```python
from build123d import *

# Parameters (mm, degrees)
F0_W     = 76.2
F0_H     = 76.2
F1_DEPTH = 584.2
F3_DEPTH = 38.1
F4_W     = 38.1
F4_H     = 38.1
F5_DEPTH = 38.1
F6_W     = 25.4
F6_H     = 114.3
F7_DEPTH = 76.201


with BuildPart() as f1:
    # F0 (on Top) → F1 (new body)
    with BuildSketch(Plane.XY):
        Rectangle(F0_W, F0_H)
    extrude(amount=F1_DEPTH)

    # F2 (on face) → F3 (join)
    with BuildSketch(Plane.XY.offset(584.2)):
        Polygon((-19.05, -19.05), (19.05, -19.05), (-19.05, 19.05), align=None)
        Polygon((-19.05, 19.05), (19.05, -19.05), (19.05, 19.05), align=None)
    extrude(amount=F3_DEPTH)

    # F4 (on face) → F5 (join)
    with BuildSketch(Plane(origin=(0, 0, 0), x_dir=(1, 0, 0), z_dir=(0, 0, -1))):
        Rectangle(F4_W, F4_H)
    extrude(amount=F5_DEPTH)

    # F6 (on face) → F7 (cut, through all)
    with BuildSketch(Plane(origin=(0, 38.1, 0), x_dir=(-1, 0, 0), z_dir=(0, 1, 0))):
        with Locations((0, 292.1)):
            Rectangle(F6_W, F6_H)
    extrude(amount=-F7_DEPTH, mode=Mode.SUBTRACT)


solid = f1.part
```
For this review, take the finished solid that the model builds, in its own axes (mm). A direction names the side the tool comes from. Round coordinates to 2 decimals unless told otherwise and drop trailing zeros. Order: outer loops, then holes, each group sorted by start corner. A loop starts at its lowest first (then second) coordinate and runs counter-clockwise, first axis right, second up.
Q1. We need section D-D, the plane x = -29. Give the boundary of the cut face in (y, z), plus the area to 3 significant figures.
Findings below:
outline: (-38.1, 0) - (38.1, 0) - (38.1, 584.2) - (-38.1, 584.2) - close
area: 44,500 mm2
Q2. Mouldability with a two-part tool opening along Z and no side actions: class faces 4 (the flat face through (0, 0, 622.3)), 5 (the flat face through (19.05, 0, -19)), 6 (the flat face through (-12.7, 1, 291)), 7 (the flat face through (0, 0, -38.1)) as pulls with the +Z half, pulls with the -Z half, needs draft (parallel to the pull), parting line crosses it, or undercut.
Findings below:
face 4: pulls with the +Z half
face 5: needs draft
face 6: undercut
face 7: pulls with the -Z half
Q3. Insertion check: P1, Ø11.5, axis at y = 4.5, z = -17, coming from the +X side; P2, Ø1, axis at x = -22.5, y = 6.5, coming from the -Z side; P3, Ø19, axis at y = -4.5, z = -12.5, coming from the -X side. Each pin has a flat end and moves straight along its axis. Give the tip position at first contact, or say it passes through.
Findings below:
P1: stops at x = 19.05
P2: stops at z = 0
P3: stops at x = -19.05
Q4. We need section C-C, the plane y = 5.5. Give the boundary of the cut face in (x, z).
Findings below:
outline: (-38.1, 0) - (-19.05, 0) - (-19.05, -38.1) - (19.05, -38.1) - (19.05, 0) - (38.1, 0) - (38.1, 584.2) - (19.05, 584.2) - (19.05, 622.3) - (-19.05, 622.3) - (-19.05, 584.2) - (-38.1, 584.2) - close; hole (-12.7, 234.95) - (12.7, 234.95) - (12.7, 349.25) - (-12.7, 349.25) - close
Q5. We need section A-A, the plane x = 3. Give the boundary of the cut face in (y, z), plus the area to 3 significant figures.
Findings below:
outline: (-38.1, 0) - (-19.05, 0) - (-19.05, -38.1) - (19.05, -38.1) - (19.05, 0) - (38.1, 0) - (38.1, 234.95) - (-38.1, 234.95) - close; (-38.1, 349.25) - (38.1, 349.25) - (38.1, 584.2) - (19.05, 584.2) - (19.05, 622.3) - (-19.05, 622.3) - (-19.05, 584.2) - (-38.1, 584.2) - close
area: 38,700 mm2
Q6. We need section B-B, the plane y = -27. Give the boundary of the cut face in (x, z).
Findings below:
outline: (-38.1, 0) - (38.1, 0) - (38.1, 584.2) - (-38.1, 584.2) - close; hole (-12.7, 234.95) - (12.7, 234.95) - (12.7, 349.25) - (-12.7, 349.25) - close
Q7. Wall thickness on line 1 (Z direction, x = -12, y = -27.5); line 2 (Z direction, x = -5.5, y = 10); line 3 (X direction, y = -22, z = 312.5): over which ranges is each line inside the solid? List them lowest first.
Findings below:
line 1: z = 0 to 234.95, 349.25 to 584.2
line 2: z = -38.1 to 234.95, 349.25 to 622.3
line 3: x = -38.1 to -12.7, 12.7 to 38.1
Q8. Machinability: for faces 1 (the flat face through (0, 1, 234.95)), 2 (the flat face through (0, 19.05, -19)), 3 (the flat face through (0, 19.05, 603)), which of the approach directions +Z, -Z, +X, -X, +Y, -Y give a long, thin tool a straight path to every point of the face, cutting with its end or side? Answer none if there is none.
Findings below:
face 1: +Y, -Y
face 2: -Z, +X, -X, +Y
face 3: +Z, +X, -X, +Y
